```python
from build123d import *

# Parameters (mm, degrees)
F0_R            = 63.5
F0_R_2          = 12.7
F2_DEPTH        = 3.81
F1_W            = 25.4
F1_H            = 3.81
F3_DEPTH        = 12.7
F3_COPIES_COUNT = 9


# Not quite as in the source:
# - a pattern or mirror of a feature is missing from the dataset's text; its kind, count and spacing are read off the source's solid


with BuildPart() as f2:
    # F0 (on Top) → F2 (new body, symmetric)
    with BuildSketch(Plane.XY):
        Circle(F0_R)
        Circle(F0_R_2, mode=Mode.SUBTRACT)
    extrude(amount=F2_DEPTH, both=True)

    # F1 (on Top) → F3 (join, symmetric)
    with BuildSketch(Plane.XY):
        with Locations((-63.5, 1.905)):
            Rectangle(F1_W, F1_H)
        with Locations((-63.5, -1.905)):
            Rectangle(F1_W, F1_H)
    f3 = extrude(amount=F3_DEPTH, both=True)

    # F3_copies: F3 ×9 about axis
    f3_copies_axis = Axis((0, 0, 0), (0, 0, 1))
    for i in range(1, F3_COPIES_COUNT):
        add(f3.rotate(f3_copies_axis, i * 360 / F3_COPIES_COUNT))


solid = f2.part
```
Model file for the job. Use its own axes, mm. A direction names the side the tool comes from. Coordinates: 2 decimals unless noted, no trailing zeros. Loops run counter-clockwise (first coordinate to the right, second up) from the corner with the lowest first, then second, coordinate; pieces in that order, holes last. Notation, with made-up numbers: (66, -26) -> (113, -26) arc R16 cw to (113, -6) -> close; hole circle Ø1 at (37.25, 7). An arc over 180 degrees is marked (long way). Answer as a JSON object with one key per item and string values.
Q1. Flat gauge pins, fed straight in: P1, Ø6, axis at y = -1.5, z = 7.5, coming from the +X side; P2, Ø1, axis at y = 11.5, z = -4, coming from the +X side; P3, Ø4, axis at y = -10.5, z = 5, coming from the +X side. Where does each tip first touch, or does it go through?
Report:
{"P1": "stops at x = -50.8", "P2": "stops at x = 62.53", "P3": "stops at x = 62.87"}
Q2. Cut at C-C (x = -43.5). List the corners of the cut face in (y, z).
Report:
{"outline": "(-46.26, -3.81) -> (-41.47, -3.81) -> (-41.47, -12.7) -> (-31.53, -12.7) -> (-31.53, -3.81) -> (31.53, -3.81) -> (31.53, -12.7) -> (41.47, -12.7) -> (41.47, -3.81) -> (46.26, -3.81) -> (46.26, 3.81) -> (41.47, 3.81) -> (41.47, 12.7) -> (31.53, 12.7) -> (31.53, 3.81) -> (-31.53, 3.81) -> (-31.53, 12.7) -> (-41.47, 12.7) -> (-41.47, 3.81) -> (-46.26, 3.81) -> close"}
Q3. Cut at A-A (y = 0). List the corners of the cut face in (x, z).
Report:
{"outline": "(-76.2, -12.7) -> (-50.8, -12.7) -> (-50.8, -3.81) -> (-12.7, -3.81) -> (-12.7, 3.81) -> (-50.8, 3.81) -> (-50.8, 12.7) -> (-76.2, 12.7) -> close; (12.7, -3.81) -> (63.5, -3.81) -> (63.5, 3.81) -> (12.7, 3.81) -> close"}
Q4. 3-axis set-ups, long thin cutter, end or side, ignore diameter. For faces 1 (the flat face through (-64, 3.81, 0)), 2 (the flat face through (47.755, -17.325, 8.317)), 3 (the flat face through (-38.881, -32.694, 8.317)), 4 (the flat face through (35.138, -53.242, 0.178)): which of +Z, -Z, +X, -X, +Y, -Y reach the whole face in a straight line?
Report:
{"face 1": "-X", "face 2": "+Z, -X", "face 3": "+Z, +X", "face 4": "+X"}
Q5. Cut at B-B (x = 0). List the corners of the cut face in (y, z), and give its area (3 significant figures).
Report:
{"outline": "(-63.5, -3.81) -> (-12.7, -3.81) -> (-12.7, 3.81) -> (-63.5, 3.81) -> close; (12.7, -3.81) -> (63.5, -3.81) -> (63.5, 3.81) -> (12.7, 3.81) -> close", "area": "774 mm2"}
Q6. Probe probe 1 along Y at (x, z) = (-53, 2.5) (3 decimals); probe 2 along Y at (x, z) = (0, 1.25); probe 3 along Z at (x, y) = (19, -40). List the from-to ranges inside material, lowest first.
Report:
{"probe 1": "y = -49.446 to -39.499, -34.975 to 34.975, 39.499 to 49.446", "probe 2": "y = -63.5 to -12.7, 12.7 to 63.5", "probe 3": "z = -3.81 to 3.81"}
Q7. Cut at D-D (y = -27). List the corners of the cut face in (x, z), and give its area (3 significant figures).
Report:
{"outline": "(-57.47, -3.81) -> (57.47, -3.81) -> (57.47, 3.81) -> (-57.47, 3.81) -> close; (63.04, -12.7) -> (71.26, -12.7) -> (71.26, 12.7) -> (63.04, 12.7) -> close", "area": "1,080 mm2"}
Q8. Pull direction Y, two halves, no side cores. Call faces 5 (the flat face through (-64, 0, -12.7)), 6 (the flat face through (-7.305, 63.372, 0.178)), 7 (the flat face through (71.586, -26.112, 0.178)), 8 (the flat face through (47.755, -17.325, -8.193)): released by +Y, released by -Y, zero draft, split by the parting line, or undercut.
Report:
{"face 5": "zero draft", "face 6": "released by +Y", "face 7": "released by -Y", "face 8": "undercut"}
